The drawing under review shows one solid part. Ordinate dimensions are in mm from its lowest x, y, z. Give positions to 0.01 mm unless a question says otherwise; leave off trailing zeros. Write each loop counter-clockwise with the first axis right and the second up, starting at its lowest first coordinate (ties: lowest second). Pieces come first, ordered by that corner, then holes. Notation, with made-up numbers: M 73.25,83.5 L 85.25,83.5 A35 cw 85.25,121.5 Z; hole C 42.5,53.25 d5. An arc over 180 degrees is marked long. Use one line per item in the form item = value. Start each with the question number.
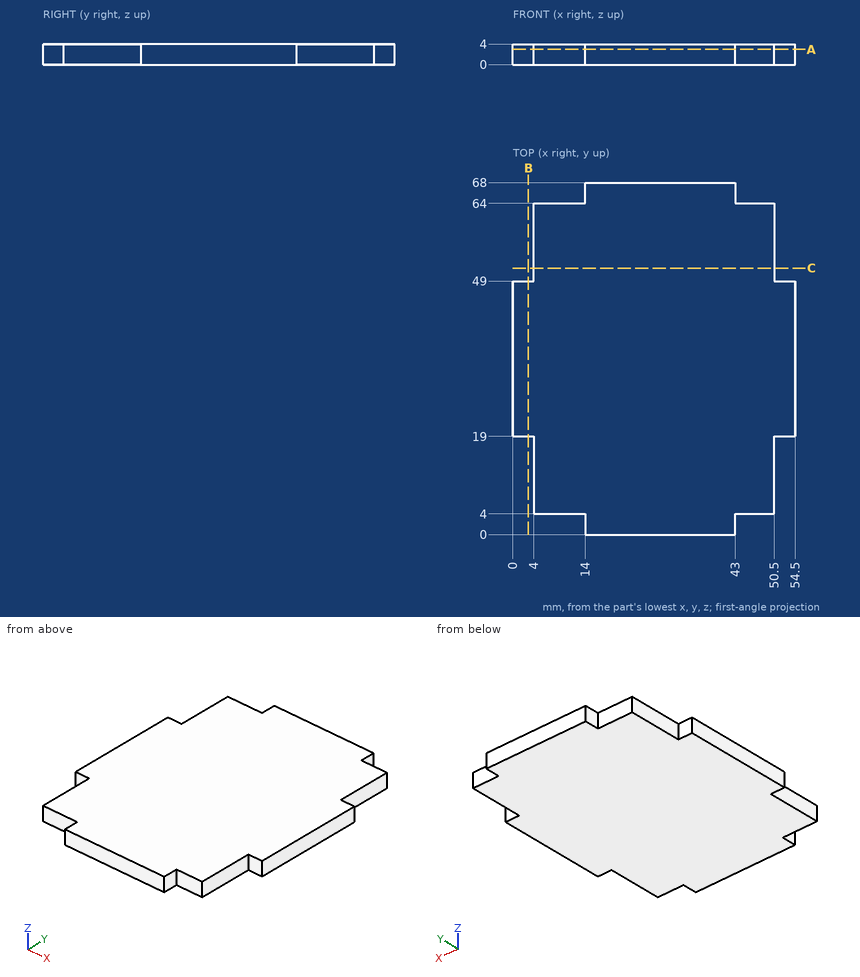
1. We need section A-A (z = 2.95). State the section outline as (x, y) points.
2. To check wall thickness, follow L1, parallel to X at y = 59, z = 1.9; L2, parallel to Y at x = 46, z = 0.2. State the ranges of each line that lie inside material, in increasing order.
3. We need section C-C (y = 51.5). State the section outline as (x, z) points.
4. Clearance check with flat-ended pins moving along their axes: pin 1 Ø2 at (y, z) = (29, 0.5) entering from -X; pin 2 Ø1.2 at (y, z) = (1.5, 2) entering from +X; pin 3 Ø2 at (y, z) = (66.5, 2) entering from -X; pin 4 Ø2 at (x, z) = (9.5, 2) entering from +Y. State where each tip first meets the part, or that it passes through.
5. We need section B-B (x = 3). State the section outline as (y, z) points.
Answer block:
q1.outline = M 0,19 L 4,19 L 4,4 L 14,4 L 14,0 L 43,0 L 43,4 L 50.5,4 L 50.5,19 L 54.5,19 L 54.5,49 L 50.5,49 L 50.5,64 L 43,64 L 43,68 L 14,68 L 14,64 L 4,64 L 4,49 L 0,49 Z
q2.L1 = 4 to 50.5
q2.L2 = 4 to 64
q3.outline = M 4,0 L 50.5,0 L 50.5,4 L 4,4 Z
q4.pin_1 = 0
q4.pin_2 = 43
q4.pin_3 = 14
q4.pin_4 = 64
q5.outline = M 19,0 L 49,0 L 49,4 L 19,4 Z
